Build history of the part. All positions in model axes, mm. Face numbers are marked on the shaded views. A direction names the side the tool comes from. Give positions to 0.01 mm unless a question says otherwise; leave off trailing zeros. Order: outer loops, then holes, each group sorted by start corner. A loop starts at its lowest first (then second) coordinate and runs counter-clockwise, first axis right, second up. Notation, with made-up numbers: (-34, 47) -> (-11, 47) arc R17 cw to (-11, 69) -> close; hole circle Ø3 at (44, 36.25). An arc over 180 degrees is marked (long way). One line per question, with ' | ' between items. Start each with the question number.
(1) Pull direction Y, two halves, no side cores. Call the marked faces 3, 4 and 5: +Y half, -Y half, draft (parallel to the pull), parting line (faces both ways), or undercut.
(2) Cut at A-A (y = 0). Give the cut face in (x, z), then the cut area to 3 significant figures.
(3) Cut at D-D (z = 6). Give the cut face in (x, y), then the cut area to 3 significant figures.
(4) Cut at B-B (z = 12.5). Give the cut face in (x, y).
(5) Cut at C-C (x = 1.9). Give the cut face in (y, z).
(6) Pin check, flat tips, straight feed: pin 1 Ø2 at (x, z) = (0, 9.5) entering from +Y; pin 2 Ø1.6 at (y, z) = (0.5, 14) entering from -X. Stop position of each tip, or through.
(7) Which spindle directions (+Z, -Z, +X, -X, +Y, -Y) get a long thin tool onto all of the face, cutting with end or side? Do the marked faces 1 and 2. Say none if no direction does.
(8) Drill centre lines: L1, parallel to Z at x = 0.85, y = -0.4; L2, parallel to Z at x = -1.75, y = -0.5; L3, parallel to Y at x = -0.15, z = 13.75. Where is each one in solid material? Low to high. Write a range as from..to.
from build123d import *

# Parameters (mm, degrees)
F3_DEPTH = 1.5
F4_SIZE  = 0.25


with BuildPart() as f1:
    # F0 (on Front) → F1 (revolve)
    with BuildSketch(Plane.XZ):
        Polygon((-1.5, 0), (0, 0), (0, 15), (-2.75, 15), (-2.75, 12), (-1.5, 12), align=None)
    revolve(axis=Axis((0, 0, -2.50989), (0, 0, -1)))

    # F2 (on face) → F3 (cut)
    with BuildSketch(Plane.XY.offset(15)):
        Polygon((-1.25, 0.721688), (-1.25, -0.721688), (0, -1.443376), (1.25, -0.721688), (1.25, 0.721688), (0, 1.443376), align=None)
    extrude(amount=-F3_DEPTH, mode=Mode.SUBTRACT)

    # F4
    f4_edges = [f1.edges().sort_by_distance(p)[0] for p in [
        (1.5, 0, 0),
    ]]
    chamfer(f4_edges, length=F4_SIZE)


solid = f1.part
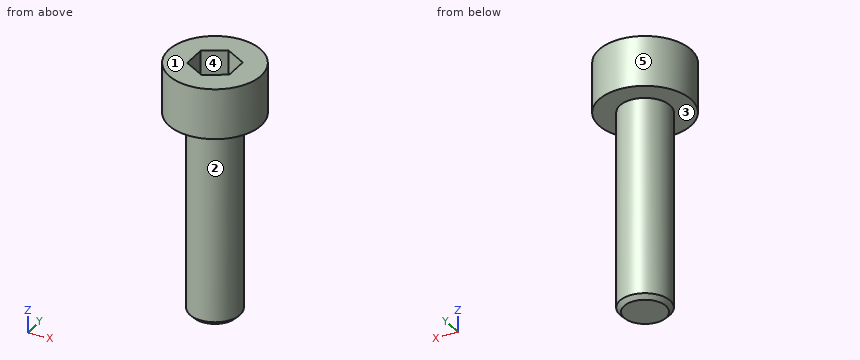
Result set:
1) face 3: draft | face 4: undercut | face 5: parting line
2) outline: (-2.75, 12) -> (-1.5, 12) -> (-1.5, 0.25) -> (-1.25, 0) -> (1.25, 0) -> (1.5, 0.25) -> (1.5, 12) -> (2.75, 12) -> (2.75, 15) -> (1.25, 15) -> (1.25, 13.5) -> (-1.25, 13.5) -> (-1.25, 15) -> (-2.75, 15) -> close | area: 48.7 mm2
3) outline: circle Ø3 at (0, 0) | area: 7.07 mm2
4) outline: circle Ø5.5 at (0, 0)
5) outline: (-1.99, 12) -> (1.99, 12) -> (1.99, 15) -> (-1.99, 15) -> close
6) pin 1: stops at y = 1.5 | pin 2: stops at x = -2.75
7) face 1: +Z, +X, -X, +Y, -Y | face 2: -Z
8) L1: z = 0..13.5 | L2: z = 12..15 | L3: y = -2.75..-1.36, 1.36..2.75
